The model under review builds one solid part; all positions refer to its coordinate system, in mm. Face numbers are marked on the shaded views. A direction names the side the tool comes from. Round coordinates to 2 decimals unless told otherwise and drop trailing zeros. Write each loop counter-clockwise with the first axis right and the second up, starting at its lowest first coordinate (ties: lowest second). Pieces come first, ordered by that corner, then holes. Notation, with made-up numbers: (44.5, 60) -> (48.5, 60) arc R31 cw to (48.5, 86) -> close; hole circle Ø7 at (76.25, 7.5). An arc over 180 degrees is marked (long way). Return JSON: item names as keys, results as strings. Group by question number.
1. Mouldability with a two-part tool opening along X and no side actions: class the marked faces 3, 4, 5 and 6 as pulls with the +X half, pulls with the -X half, needs draft (parallel to the pull), parting line crosses it, or undercut.
2. Take a section at C-C, the plane z = 18.5. Write out the cut boundary in (x, y).
3. Take a section at A-A, the plane z = 32.5. Write out the cut boundary in (x, y).
4. Clearance check with flat-ended pins moving along their axes: P1, Ø2, axis at x = -79, z = 29.5, coming from the +Y side; P2, Ø1, axis at x = -68, y = 21.5, coming from the +Z side. State where each tip first meets the part, or that it passes through.
5. Take a section at B-B, the plane x = -95. Write out the cut boundary in (y, z).
6. For line 1 along X through (y, z) = (-8, 18.5); line 2 along X through (y, z) = (-4.5, 8); line 3 along Y through (x, z) = (-95, 19.5), list the stretches that pass through material, from the lowest coordinate up. Write a range as from..to.
7. Take a section at D-D, the plane y = 24.5. Write out the cut boundary in (x, z), then the cut area to 3 significant figures.
8. Tool access review of the marked faces 1 and 2: name each direction out of +Z, -Z, +X, -X, +Y, -Y from which nothing blocks a thin tool from reaching the whole face with its end or side.
from build123d import *

# Parameters (mm, degrees)
BOSS_EXTRUDE1_DEPTH     = 38
SKETCH3_R               = 10
BOSS_EXTRUDE4_DEPTH     = 84
CUT_EXTRUDE1_DEPTH      = 142.830361505
CUT_EXTRUDE1_DEPTH_BACK = 142.830361505
SKETCH4_R               = 8
CUT_EXTRUDE2_DEPTH      = 142.830361505
CUT_EXTRUDE2_DEPTH_BACK = 142.830361505
BOSS_EXTRUDE5_START     = -16
BOSS_EXTRUDE5_DEPTH     = 52


with BuildPart() as part:
    # Sketch2 → Boss-Extrude1 (new body)
    with BuildSketch(Plane.XY):
        Polygon((-107.776859504, 29.566115702), (-69.776859504, 29.566115702), (-69.776859504, 45.066115702), (-49.776859504, 45.066115702), (-49.776859504, -38.933884298), (-69.776859504, -38.933884298), (-69.776859504, -23.433884298), (-107.776859504, -23.433884298), align=None)
    extrude(amount=BOSS_EXTRUDE1_DEPTH)

    # Sketch3 → Boss-Extrude4 (add)
    with BuildSketch(Plane(origin=(0, 45.066115702, 0), x_dir=(1, 0, 0), z_dir=(0, 1, 0))):
        with Locations((-62.776859504, -18.5)):
            Circle(SKETCH3_R)
    extrude(amount=-BOSS_EXTRUDE4_DEPTH)

    # Sketch4 → Cut-Extrude1 (cut, two sides: drawn at the far end of the back side and taken through both)
    with BuildSketch(Plane(origin=(0, 45.066115702, 0), x_dir=(1, 0, 0), z_dir=(0, 1, 0)).offset(-CUT_EXTRUDE1_DEPTH_BACK)):
        with Locations(Location((-62.776859504, -18.5, 0), (0, 0, 270))):
            Circle(SKETCH4_R)
    extrude(amount=CUT_EXTRUDE1_DEPTH + CUT_EXTRUDE1_DEPTH_BACK, mode=Mode.SUBTRACT)

    # Sketch5 → Cut-Extrude2 (cut, two sides: drawn at the far end of the back side and taken through both)
    with BuildSketch(Plane(origin=(0, 45.066115702, 0), x_dir=(1, 0, 0), z_dir=(0, 1, 0)).offset(-CUT_EXTRUDE2_DEPTH_BACK)):
        with BuildLine():
            Line((-56.443650173, 0), (-69.776859504, 0))
            Line((-69.776859504, 0), (-69.776859504, -11.358571571))
            ThreePointArc((-69.776859504, -11.358571571), (-52.776859504, -18.5), (-69.776859504, -25.641428429))
            Line((-69.776859504, -25.641428429), (-69.776859504, -38))
            Line((-69.776859504, -38), (-56.443650173, -38))
            Line((-56.443650173, -38), (-49.776859504, -38))
            Line((-49.776859504, -38), (-49.776859504, 0))
            Line((-49.776859504, 0), (-56.443650173, 0))
        make_face()
    extrude(amount=CUT_EXTRUDE2_DEPTH + CUT_EXTRUDE2_DEPTH_BACK, mode=Mode.SUBTRACT)

    # Sketch6 → Boss-Extrude5 (add)
    with BuildSketch(Plane(origin=(0, 45.066115702, 0), x_dir=(1, 0, 0), z_dir=(0, 1, 0)).offset(BOSS_EXTRUDE5_START)):
        with BuildLine():
            Line((-57.850011392, 0), (-52.785705753, 0))
            Line((-52.785705753, 0), (-51.650992669, 0))
            Line((-51.650992669, 0), (-51.650992669, -38))
            Line((-51.650992669, -38), (-52.785705753, -38))
            Line((-52.785705753, -38), (-57.850011392, -38))
            Line((-57.850011392, -38), (-57.850011392, -24.802869797))
            ThreePointArc((-57.850011392, -24.802869797), (-54.776859504, -18.5), (-57.850011392, -12.197130203))
            Line((-57.850011392, -12.197130203), (-57.850011392, 0))
        make_face()
    extrude(amount=-BOSS_EXTRUDE5_DEPTH)


solid = part.part
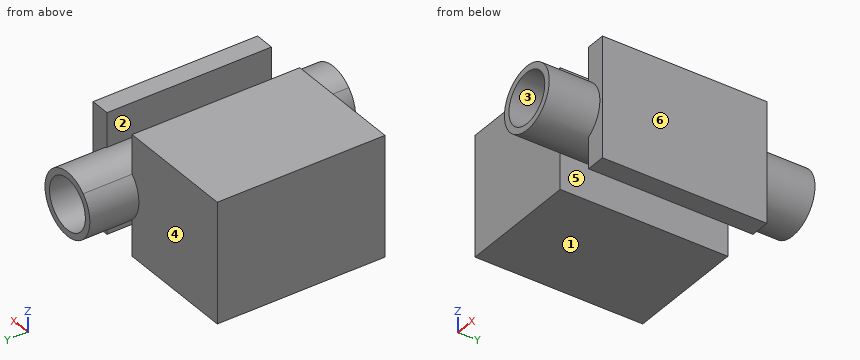
Output:
{
 "1": {"face 3": "undercut", "face 4": "needs draft", "face 5": "undercut", "face 6": "pulls with the +X half"},
 "2": {"outline": "(-107.78, -23.43) -> (-72.78, -23.43) -> (-72.78, -38.93) -> (-70.78, -38.93) -> (-70.78, 45.07) -> (-72.78, 45.07) -> (-72.78, 29.57) -> (-107.78, 29.57) -> close; (-54.78, -38.93) -> (-52.78, -38.93) -> (-52.78, -22.93) -> (-51.65, -22.93) -> (-51.65, 29.07) -> (-52.78, 29.07) -> (-52.78, 45.07) -> (-54.78, 45.07) -> close"},
 "3": {"outline": "(-107.78, -23.43) -> (-69.78, -23.43) -> (-69.78, 29.57) -> (-107.78, 29.57) -> close; (-57.85, -22.93) -> (-51.65, -22.93) -> (-51.65, 29.07) -> (-57.85, 29.07) -> close"},
 "4": {"P1": "stops at y = 29.57", "P2": "stops at z = 27.31"},
 "5": {"outline": "(-23.43, 0) -> (29.57, 0) -> (29.57, 38) -> (-23.43, 38) -> close"},
 "6": {"line 1": "x = -107.78..-70.78, -54.78..-51.65", "line 2": "x = -107.78..-69.78, -57.85..-51.65", "line 3": "y = -23.43..29.57"},
 "7": {"outline": "(-107.78, 0) -> (-69.78, 0) -> (-69.78, 11.36) arc R10 ccw to (-57.85, 9.8) -> (-57.85, 0) -> (-51.65, 0) -> (-51.65, 38) -> (-57.85, 38) -> (-57.85, 27.2) arc R10 ccw to (-69.78, 25.64) -> (-69.78, 38) -> (-107.78, 38) -> close; hole circle Ø16 at (-62.78, 18.5)", "area": "1,700 mm^2"},
 "8": {"face 1": "-Z, +X, -X, +Y, -Y", "face 2": "+Z, +Y, -Y"}
}
